Source: CAD feature listing. Evaluate the final solid. Frame: model axes, mm. A direction names the side the tool comes from. Give positions to 0.01 mm unless a question says otherwise; leave off trailing zeros. Loops run counter-clockwise (first coordinate to the right, second up) from the corner with the lowest first, then second, coordinate; pieces in that order, holes last. Notation, with made-up numbers: M 6.25,-37 L 41.25,-37 A24 cw 41.25,-1 Z; hole C 89,-36.75 d10. An arc over 180 degrees is marked long. Put each result on its own line as item: value.
from build123d import *

# Parameters (mm, degrees)
F0_W     = 12.7
F0_H     = 233.4768
F1_DEPTH = 6.35


# Not quite as in the source:
# - a feature names something its author has since deleted; it is built from what else it names


with BuildPart() as f1:
    # F0 (on Top) → F1 (new body)
    with BuildSketch(Plane.XY):
        Polygon((88.9, -116.7384), (76.2, -116.7384), (-76.2, -116.7384), (-101.6, -116.7384), (-101.6, -142.1384), (101.6, -142.1384), (101.6, -116.7384), align=None)
        Polygon((-76.2, 116.7384), (76.2, 116.7384), (88.9, 116.7384), (101.6, 116.7384), (101.6, 142.1384), (-101.6, 142.1384), (-101.6, 116.7384), align=None)
        with Locations((95.25, 0)):
            Rectangle(F0_W, F0_H)
        with Locations((82.55, 0)):
            Rectangle(F0_W, F0_H)
    extrude(amount=F1_DEPTH)


solid = f1.part
1. Section query C-C (y = 49). Output: boundary loops of the cut face in (x, z), plus the area to 3 significant figures.
Found:
outline: M 76.2,0 L 101.6,0 L 101.6,6.35 L 76.2,6.35 Z
area: 161 mm^2
2. Contact query for a flat-ended pin moving along its axis: P1, Ø1.9, axis at y = -10, z = 2, coming from the -X side. Output: stop coordinate, or through.
Found:
P1: x = 76.2
3. Access query for faces 4 (the flat face through (101.6, -2, 3)), 5 (the flat face through (76.2, -2, 3)). Directions: +Z, -Z, +X, -X, +Y, -Y. A direction counts if a zero-diameter tool reaches every point of the face in a straight line with its end or side. Return the directions, or none.
Found:
face 4: +Z, -Z, +X, +Y, -Y
face 5: +Z, -Z, -X
4. Section query A-A (x = 66.5). Output: boundary loops of the cut face in (y, z).
Found:
outline: M -142.14,0 L -116.74,0 L -116.74,6.35 L -142.14,6.35 Z; M 116.74,0 L 142.14,0 L 142.14,6.35 L 116.74,6.35 Z
5. Section query B-B (z = 5.25). Output: boundary loops of the cut face in (x, y).
Found:
outline: M -101.6,-142.14 L 101.6,-142.14 L 101.6,142.14 L -101.6,142.14 L -101.6,116.74 L 76.2,116.74 L 76.2,-116.74 L -101.6,-116.74 Z
6. Material intervals for line 1 (Y direction, x = 2, z = 1.5); line 2 (X direction, y = -71, z = 3.75), sorted ascending. Write a range as from..to.
Found:
line 1: -142.14..-116.74, 116.74..142.14
line 2: 76.2..101.6
7. Draft query along Y for faces 1 (the flat face through (82, 11, 0)), 2 (the flat face through (-1, -142.138, 3)), 3 (the flat face through (-11, -116.738, 3)). Return one class per face: pulls with the +Y half, pulls with the -Y half, needs draft (parallel to the pull), parting line crosses it, or undercut.
Found:
face 1: needs draft
face 2: pulls with the -Y half
face 3: undercut
